For this review, take the finished solid that the model builds, in its own axes (mm). A direction names the side the tool comes from. Coordinates: 2 decimals unless noted, no trailing zeros. Order: outer loops, then holes, each group sorted by start corner. A loop starts at its lowest first (then second) coordinate and runs counter-clockwise, first axis right, second up.
from build123d import *

# Parameters (mm, degrees)
SKETCH1_W              = 25.4
SKETCH1_H              = 25.4
SKETCH1_W_2            = 19.05
SKETCH1_H_2            = 19.05
BOSS_EXTRUDE1_DEPTH    = 407.19375
F_10_CLEARANCE_HOLE1_D = 5.1054
CUT_EXTRUDE1_REACH     = 410.183
SKETCH4_R              = 7.62


with BuildPart() as part:
    # Sketch1 → Boss-Extrude1 (new body)
    with BuildSketch(Plane.XY):
        Rectangle(SKETCH1_W, SKETCH1_H)
        Rectangle(SKETCH1_W_2, SKETCH1_H_2, mode=Mode.SUBTRACT)
    extrude(amount=BOSS_EXTRUDE1_DEPTH)

    # #10 Clearance Hole1 (through all)
    with Locations(Plane(origin=(146.05, 12.7, 546.735), x_dir=(0, 0, 1), z_dir=(0, 1, 0))):
        with Locations((-423.545, -146.05), (-262.255, -146.05)):
            Hole(F_10_CLEARANCE_HOLE1_D / 2)

    # Sketch4 → Cut-Extrude1 (cut, up to next)
    with BuildSketch(Plane(origin=(0, -12.7, 0), x_dir=(1, 0, 0), z_dir=(0, 1, 0)), mode=Mode.PRIVATE) as cut_extrude1_sk1:
        with Locations(Location((0, -123.19, 0), (0, 0, 90))):
            Circle(SKETCH4_R)
    cut_extrude1_tool1 = extrude(cut_extrude1_sk1.sketch, amount=CUT_EXTRUDE1_REACH, mode=Mode.PRIVATE) & part.part
    # Sketch4 → Cut-Extrude1 (cut, up to next)
    with BuildSketch(Plane(origin=(0, -12.7, 0), x_dir=(1, 0, 0), z_dir=(0, 1, 0)), mode=Mode.PRIVATE) as cut_extrude1_sk2:
        with Locations(Location((0, -284.48, 0), (0, 0, 90))):
            Circle(SKETCH4_R)
    cut_extrude1_tool2 = extrude(cut_extrude1_sk2.sketch, amount=CUT_EXTRUDE1_REACH, mode=Mode.PRIVATE) & part.part
    add(cut_extrude1_tool1.solids().sort_by_distance((0, -12.7, 123.19))[0], mode=Mode.SUBTRACT)
    add(cut_extrude1_tool2.solids().sort_by_distance((0, -12.7, 284.48))[0], mode=Mode.SUBTRACT)


solid = part.part
1. Machinability: for faces 1 (the face through (-5.15, -11.135, 128.806)), 2 (the face through (0, -9.525, 201)), 3 (the face through (-12.7, 0, 201)), which of the approach directions +Z, -Z, +X, -X, +Y, -Y give a long, thin tool a straight path to every point of the face, cutting with its end or side? Answer none if there is none.
Answer below:
face 1: -Y
face 2: +Z, -Z
face 3: +Z, -Z, -X, +Y, -Y
2. Take a section at A-A, the plane y = 1.25. Give the boundary of the cut face in (x, z) (3 decimals).
Answer below:
outline: (-12.7, 0) - (-9.525, 0) - (-9.525, 407.194) - (-12.7, 407.194) - close; (9.525, 0) - (12.7, 0) - (12.7, 407.194) - (9.525, 407.194) - close
3. Clearance check with a flat-ended pin moving along its axis: pin 1 Ø6 at (x, z) = (0, 284.48) entering from -Y (3 decimals). State where the tip first meets the part, or that it passes through.
Answer below:
pin 1: stops at y = 9.525
4. To check wall thickness, follow L1, parallel to Y at x = -0.5, z = 193 (3 decimals); L2, parallel to X at y = -10.6, z = 284.48. State the ranges of each line that lie inside material, in increasing order.
Answer below:
L1: y = -12.7 to -9.525, 9.525 to 12.7
L2: x = -12.7 to -7.62, 7.62 to 12.7
5. The part is to be moulded in two halves that separate along Y. For faces 4 (the face through (0, -12.7, 201)), 5 (the face through (-9.525, 0, 201)), 6 (the face through (0, 9.525, 201)), 7 (the face through (12.7, 0, 201)), say which applies: +Y half, -Y half, draft (parallel to the pull), parting line (faces both ways), or undercut.
Answer below:
face 4: -Y half
face 5: undercut
face 6: undercut
face 7: draft
6. Take a section at B-B, the plane z = 376. Give the boundary of the cut face in (x, y) (3 decimals), plus the area to 3 significant figures.
Answer below:
outline: (-12.7, -12.7) - (12.7, -12.7) - (12.7, 12.7) - (-12.7, 12.7) - close; hole (-9.525, -9.525) - (9.525, -9.525) - (9.525, 9.525) - (-9.525, 9.525) - close
area: 282 mm2
